```python
from build123d import *

# Parameters (mm, degrees)
BOSS_EXTRUDE1_DEPTH       = 12.7
F_8_CLEARANCE_HOLE1_D     = 4.4958
F_8_CLEARANCE_HOLE1_DEPTH = 61.468
F_8_CLEARANCE_HOLE1_TIP   = 1.350674586


with BuildPart() as part:
    # Sketch2 → Boss-Extrude1 (new body)
    with BuildSketch(Plane.XY):
        with BuildLine():
            Line((12.5, 0), (22.616843834, 0))
            Line((22.616843834, 0), (22.616843834, 3.175))
            Line((22.616843834, 3.175), (16.266843834, 3.175))
            Line((16.266843834, 3.175), (9.04996547, 15.675))
            Line((9.04996547, 15.675), (-9.04996547, 15.675))
            Line((-9.04996547, 15.675), (-16.266843834, 3.175))
            Line((-16.266843834, 3.175), (-22.616843834, 3.175))
            Line((-22.616843834, 3.175), (-22.616843834, 0))
            Line((-22.616843834, 0), (-12.5, 0))
            ThreePointArc((-12.5, 0), (0, 12.5), (12.5, 0))
        make_face()
    extrude(amount=BOSS_EXTRUDE1_DEPTH)

    # #8 Clearance Hole1
    with Locations(Plane(origin=(0, 3.175, 0), x_dir=(1, 0, 0), z_dir=(0, 1, 0))):
        with Locations((19.441843834, -6.35), (-19.441843834, -6.35)):
            Hole(F_8_CLEARANCE_HOLE1_D / 2, depth=F_8_CLEARANCE_HOLE1_DEPTH)
            with Locations((0, 0, -(F_8_CLEARANCE_HOLE1_DEPTH + F_8_CLEARANCE_HOLE1_TIP / 2))):  # 118° drill point
                Cone(0, F_8_CLEARANCE_HOLE1_D / 2, F_8_CLEARANCE_HOLE1_TIP, mode=Mode.SUBTRACT)


solid = part.part
```
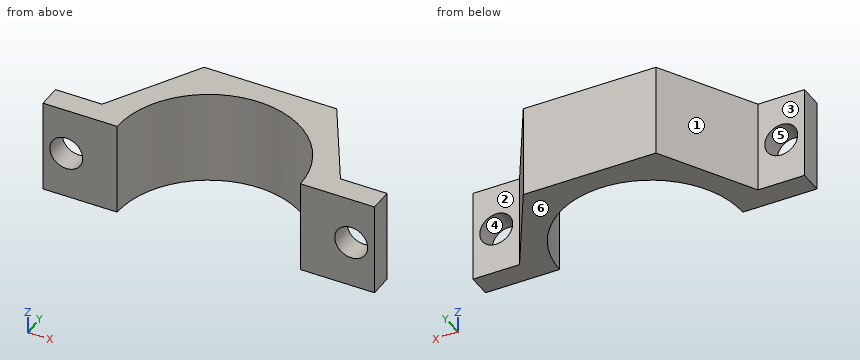
Input: part model. Units: mm. Frame: model coordinates. Face numbers are marked on the shaded views. A direction names the side the tool comes from. Coordinates: 2 decimals unless noted, no trailing zeros. Loops run counter-clockwise (first coordinate to the right, second up) from the corner with the lowest first, then second, coordinate; pieces in that order, holes last. Notation, with made-up numbers: M 8,33 L 19,33 A14 ccw 19,44 Z; hole C -31,24.5 d4. An arc over 180 degrees is marked long. Answer in a Markdown table with one row per item.
1. Section B-B, the plane y = 2. Output: boundary loops of the cut face in (x, z).
Response:
| item | result |
|---|---|
| outline | M -22.62,0 L -12.34,0 L -12.34,12.7 L -22.62,12.7 Z; M 12.34,0 L 22.62,0 L 22.62,12.7 L 12.34,12.7 Z; hole C -19.44,6.35 d4.5; hole C 19.44,6.35 d4.5 |
2. First-contact query: pin 1 (3 mm diameter, centred on x = 21, z = 7.5, fed in from +Y) (3 decimals); pin 2 (5 mm diameter, centred on x = -3.5, y = 11.5, fed in from -Z); pin 3 (2 mm diameter, centred on x = -5.5, z = 4.5, fed in from -Y); pin 4 (2 mm diameter, centred on y = 6.5, z = 8.5, fed in from +X). Flat tips, straight axial feed; report the tip coordinate or a pass-through.
Response:
| item | result |
|---|---|
| pin 1 | stops at y = 3.175 |
| pin 2 | stops at z = 0 |
| pin 3 | stops at y = 10.68 |
| pin 4 | stops at x = 14.92 |
3. Draft query along Z for the marked faces 3, 4, 5 and 6. Return one class per face: pulls with the +Z half, pulls with the -Z half, needs draft (parallel to the pull), parting line crosses it, or undercut.
Response:
| item | result |
|---|---|
| face 3 | needs draft |
| face 4 | undercut |
| face 5 | undercut |
| face 6 | pulls with the -Z half |
4. Section A-A, the plane z = 6.35. Output: boundary loops of the cut face in (x, y) (3 decimals), then the cut area to 3 significant figures.
Response:
| item | result |
|---|---|
| outline | M -22.617,0 L -21.69,0 L -21.69,3.175 L -22.617,3.175 Z; M -17.194,0 L -12.5,0 A12.5 cw 12.5,0 L 17.194,0 L 17.194,3.175 L 16.267,3.175 L 9.05,15.675 L -9.05,15.675 L -16.267,3.175 L -17.194,3.175 Z; M 21.69,0 L 22.617,0 L 22.617,3.175 L 21.69,3.175 Z |
| area | 186 mm2 |
5. Section D-D, the plane z = 11.25. Output: boundary loops of the cut face in (x, y) (3 decimals), then the cut area to 3 significant figures.
Response:
| item | result |
|---|---|
| outline | M -22.617,0 L -12.5,0 A12.5 cw 12.5,0 L 22.617,0 L 22.617,3.175 L 16.267,3.175 L 9.05,15.675 L -9.05,15.675 L -16.267,3.175 L -22.617,3.175 Z |
| area | 215 mm2 |
6. Material intervals for line 1 (Z direction, x = -19.5, y = 2.75); line 2 (X direction, y = 1, z = 6.5); line 3 (X direction, y = 4, z = 2.75), sorted ascending.
Response:
| item | result |
|---|---|
| line 1 | z = 0 to 4.1, 8.6 to 12.7 |
| line 2 | x = -22.62 to -21.68, -17.2 to -12.46, 12.46 to 17.2, 21.68 to 22.62 |
| line 3 | x = -15.79 to -11.84, 11.84 to 15.79 |
7. Section C-C, the plane y = 6. Output: boundary loops of the cut face in (x, z), then the cut area to 3 significant figures.
Response:
| item | result |
|---|---|
| outline | M -14.64,0 L -10.97,0 L -10.97,12.7 L -14.64,12.7 Z; M 10.97,0 L 14.64,0 L 14.64,12.7 L 10.97,12.7 Z |
| area | 93.2 mm2 |
8. Reachability of the marked faces 1 and 2 from +Z, -Z, +X, -X, +Y, -Y: full face, straight path, thin tool, end or side. Return the list, or none.
Response:
| item | result |
|---|---|
| face 1 | +Z, -Z, -X, +Y |
| face 2 | +Z, -Z, +X, +Y |
